```python
from build123d import *

# Parameters (mm, degrees)
SKETCH8_R           = 11.15
BOSS_EXTRUDE4_DEPTH = 3
BOSS_EXTRUDE5_DEPTH = 12
SKETCH11_R          = 3.25
CUT_EXTRUDE3_DEPTH  = 13.2
SKETCH14_R          = 1.7
CUT_EXTRUDE4_DEPTH  = 17.684550296
FILLET1_R           = 8.5


with BuildPart() as part:
    # Sketch8 → Boss-Extrude4 (new body)
    with BuildSketch(Plane(origin=(0, 0, 0), x_dir=(1, 0, 0), z_dir=(0, 1, 0))):
        with BuildLine():
            Line((-35.85, -6), (-29.521443478, -6))
            ThreePointArc((-29.521443478, -6), (0, -30.125), (29.521443478, -6))
            Line((29.521443478, -6), (35.85, -6))
            Line((35.85, -6), (35.85, 6))
            Line((35.85, 6), (29.521443478, 6))
            ThreePointArc((29.521443478, 6), (0, 30.125), (-29.521443478, 6))
            Line((-29.521443478, 6), (-35.85, 6))
            Line((-35.85, 6), (-35.85, -6))
        make_face()
        Circle(SKETCH8_R, mode=Mode.SUBTRACT)
    extrude(amount=BOSS_EXTRUDE4_DEPTH)

    # Sketch9 → Boss-Extrude5 (add)
    with BuildSketch(Plane.XY.offset(6)):
        Polygon((-35.85, 3), (-35.85, -64.95), (-54.85, -64.95), (-40.85, -48.265449704), (-40.85, 3), align=None)
    boss_extrude5 = extrude(amount=-BOSS_EXTRUDE5_DEPTH)

    # Sketch11 → Cut-Extrude3 (cut)
    with BuildSketch(Plane.ZX.offset(-48.265449704)):
        with Locations((0, -46.1)):
            Circle(SKETCH11_R)
    cut_extrude3 = extrude(amount=-CUT_EXTRUDE3_DEPTH, mode=Mode.SUBTRACT)

    # Sketch14 → Cut-Extrude4 (cut, through all)
    with BuildSketch(Plane.ZX.offset(-48.265449704)):
        with Locations((0, -46.1)):
            Circle(SKETCH14_R)
    cut_extrude4 = extrude(amount=-CUT_EXTRUDE4_DEPTH, mode=Mode.SUBTRACT)

    # Mirror3: Boss-Extrude5, Cut-Extrude3, Cut-Extrude4 across plane
    add(boss_extrude5.mirror(Plane(origin=(0, 0, 0), x_dir=(0, 0, 1), z_dir=(1, 0, 0))))
    add(cut_extrude3.mirror(Plane(origin=(0, 0, 0), x_dir=(0, 0, 1), z_dir=(1, 0, 0))), mode=Mode.SUBTRACT)
    add(cut_extrude4.mirror(Plane(origin=(0, 0, 0), x_dir=(0, 0, 1), z_dir=(1, 0, 0))), mode=Mode.SUBTRACT)

    # Fillet1
    fillet1_edges = [part.edges().sort_by_distance(p)[0] for p in [
        (-29.521443478, 1.5, -6),
        (29.521443478, 1.5, -6),
        (29.521443478, 1.5, 6),
        (-29.521443478, 1.5, 6),
    ]]
    fillet(fillet1_edges, radius=FILLET1_R)


solid = part.part
```
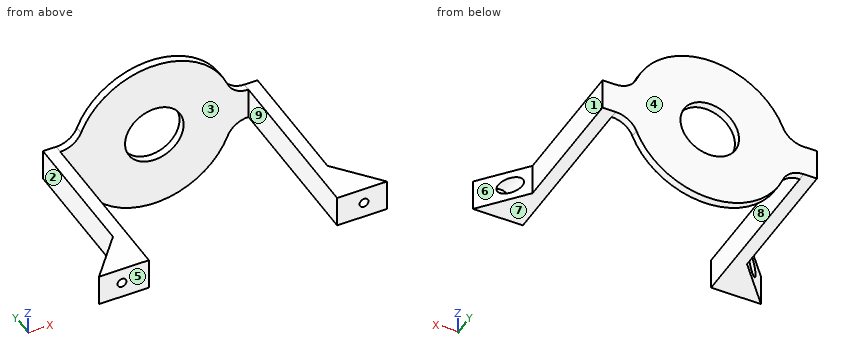
The listing builds one solid part. Answer for the finished solid, in the listing's coordinates (mm). Face numbers are marked on the shaded views. A direction names the side the tool comes from. Coordinates: 2 decimals unless noted, no trailing zeros. Loops run counter-clockwise (first coordinate to the right, second up) from the corner with the lowest first, then second, coordinate; pieces in that order, holes last. Notation, with made-up numbers: (50, 34) - (76, 34) arc R14 ccw to (76, 56) - close; hole circle Ø11 at (48, -2). An arc over 180 degrees is marked (long way). Use a Markdown table: item, result. Add a question column.
1) The part is cut by section D-D, the plane x = -46.1. Give the vertices of the cut face in (y, z), and give its area (3 significant figures).
2) The part is cut by section B-B, the plane y = -16. Give the vertices of the cut face in (x, z), and give its area (3 significant figures).
3) The part is cut by section C-C, the plane z = 0. State how many separate pieces and enclosed holes the cut face has, and give its area (3 significant figures).
4) For the marked faces 1, 2, 3, 4 and 5, determine the directions among +Z, -Z, +X, -X, +Y, -Y from which every point of the face is accessible in a straight line to the end or side of a thin tool.
5) The mould has two halves that part along X. Classify the marked faces 6, 7, 8 and 9: released by +X, released by -X, zero draft, split by the parting line, or undercut.
6) Given pin 1 (4.5 mm diameter, centred on x = 46.1, z = 0, fed in from +Y); pin 2 (8.5 mm diameter, centred on x = 46.1, z = 0, fed in from +Y); pin 3 (5 mm diameter, centred on x = -39.5, y = -9, fed in from -Z), each flat-ended and moving along its own axis, determine where each tip first touches the part or whether it passes through.
7) The part is cut by section A-A, the plane x = 0. Give the vertices of the cut face in (y, z) (3 decimals).
8) Find the intervals of material crossed by line 1 (X direction, y = -57, z = 0); line 2 (X direction, y = -25, z = -1.5); line 3 (Z direction, x = -46.1, y = -55.25), in increasing order.
Here are the results:
| question | item | result |
|---|---|---|
| 1 | outline | (-64.95, -6) - (-54.52, -6) - (-54.52, -3.25) - (-61.47, -3.25) - (-61.47, -1.7) - (-64.95, -1.7) - close; (-64.95, 1.7) - (-61.47, 1.7) - (-61.47, 3.25) - (-54.52, 3.25) - (-54.52, 6) - (-64.95, 6) - close |
| 1 | area | 68.2 mm^2 |
| 2 | outline | (-40.85, -6) - (-35.85, -6) - (-35.85, 6) - (-40.85, 6) - close; (35.85, -6) - (40.85, -6) - (40.85, 6) - (35.85, 6) - close |
| 2 | area | 120 mm^2 |
| 3 | separate pieces | 4 |
| 3 | enclosed holes | 0 |
| 3 | area | 947 mm^2 |
| 4 | face 1 | +Z, -Z, +X, +Y |
| 4 | face 2 | +Z, -Z, -X, +Y |
| 4 | face 3 | +Z, -Z, -Y |
| 4 | face 4 | +Z, -Z, +X, -X, +Y |
| 4 | face 5 | +Z, -Z, +X, -X, -Y |
| 5 | face 6 | released by +X |
| 5 | face 7 | zero draft |
| 5 | face 8 | undercut |
| 5 | face 9 | undercut |
| 6 | pin 1 | stops at y = -61.47 |
| 6 | pin 2 | stops at y = -49.46 |
| 6 | pin 3 | stops at z = -6 |
| 7 | outline | (0, -30.125) - (3, -30.125) - (3, -11.15) - (0, -11.15) - close; (0, 11.15) - (3, 11.15) - (3, 30.125) - (0, 30.125) - close |
| 8 | line 1 | x = -42.85 to -35.85, 35.85 to 42.85 |
| 8 | line 2 | x = -40.85 to -35.85, 35.85 to 40.85 |
| 8 | line 3 | z = -6 to -3.25, 3.25 to 6 |
